CAD build for the part. Positions are in the model's coordinates, mm. Face numbers are marked on the shaded views. A direction names the side the tool comes from. Give positions to 0.01 mm unless a question says otherwise; leave off trailing zeros. Order: outer loops, then holes, each group sorted by start corner. A loop starts at its lowest first (then second) coordinate and runs counter-clockwise, first axis right, second up.
Item 1: Wall check: L1, parallel to Z at x = 152, y = 4.75; L2, parallel to Z at x = 124, y = 11.25; L3, parallel to Y at x = 95, z = 6. Give the ranges that are in metal, low to high.
Item 2: Which spindle directions (+Z, -Z, +X, -X, +Y, -Y) get a long thin tool onto all of the face, cutting with end or side? Do the marked faces 1 and 2. Say none if no direction does.
Item 3: Flat gauge pins, fed straight in: P1, Ø12, axis at x = 61.5, z = -30.5, coming from the -Y side; P2, Ø13, axis at x = 152.4, z = -25.4, coming from the +Y side; P3, Ø17.5, axis at x = 76.2, z = -25.4, coming from the +Y side. Where does each tip first touch, or does it go through?
Item 4: Band-saw the part on D-D on x = 107. Give the cut face in (y, z), plus the area to 3 significant figures.
Item 5: Two-plate mould, pull along X, no slides. Class the marked faces 3, 4, 5 and 6: released by +X, released by -X, zero draft, split by the parting line, or undercut.
Item 6: Band-saw the part on B-B on y = 10. Count the separate pieces of the cut face and the enclosed holes in it, plus the area to 3 significant figures.
Item 7: Band-saw the part on A-A on x = 25.4. Give the cut face in (y, z).
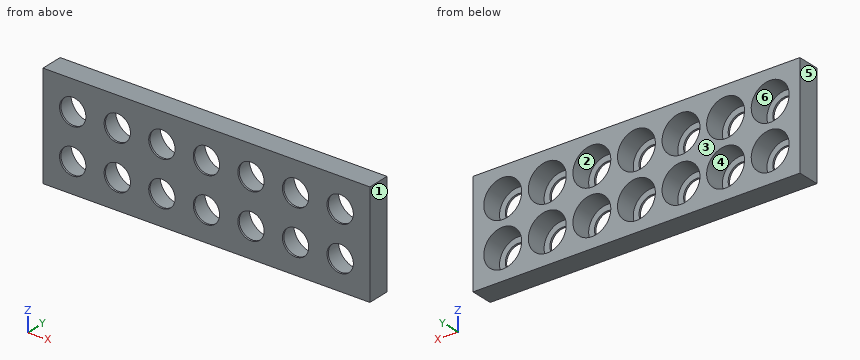
```python
from build123d import *

# Parameters (mm, degrees)
SKETCH1_W           = 186.266666666
SKETCH1_H           = 59.266666666
SKETCH1_R           = 10.8
BOSS_EXTRUDE2_DEPTH = 12.7
SKETCH1_4_R         = 10.8
SKETCH1_4_R_2       = 7.5
BOSS_EXTRUDE3_DEPTH = 1.016


with BuildPart() as part:
    # Sketch1 → Boss-Extrude2 (new body)
    with BuildSketch(Plane(origin=(0, 0, 0), x_dir=(1, 0, 0), z_dir=(0, 1, 0))):
        with Locations((76.2, 12.7)):
            Rectangle(SKETCH1_W, SKETCH1_H)
        with Locations(Location((0, 25.4, 0), (0, 0, 270))):
            Circle(SKETCH1_R, mode=Mode.SUBTRACT)
        with Locations(Location((152.4, 25.4, 0), (0, 0, 270))):
            Circle(SKETCH1_R, mode=Mode.SUBTRACT)
        with Locations(Location((127, 25.4, 0), (0, 0, 270))):
            Circle(SKETCH1_R, mode=Mode.SUBTRACT)
        with Locations(Location((101.6, 25.4, 0), (0, 0, 270))):
            Circle(SKETCH1_R, mode=Mode.SUBTRACT)
        with Locations(Location((76.2, 25.4, 0), (0, 0, 270))):
            Circle(SKETCH1_R, mode=Mode.SUBTRACT)
        with Locations(Location((50.8, 25.4, 0), (0, 0, 270))):
            Circle(SKETCH1_R, mode=Mode.SUBTRACT)
        with Locations(Location((25.4, 25.4, 0), (0, 0, 270))):
            Circle(SKETCH1_R, mode=Mode.SUBTRACT)
        with Locations(Location((152.4, 0, 0), (0, 0, 270))):
            Circle(SKETCH1_R, mode=Mode.SUBTRACT)
        with Locations(Location((127, 0, 0), (0, 0, 270))):
            Circle(SKETCH1_R, mode=Mode.SUBTRACT)
        with Locations(Location((101.6, 0, 0), (0, 0, 270))):
            Circle(SKETCH1_R, mode=Mode.SUBTRACT)
        with Locations(Location((76.2, 0, 0), (0, 0, 270))):
            Circle(SKETCH1_R, mode=Mode.SUBTRACT)
        with Locations(Location((50.8, 0, 0), (0, 0, 270))):
            Circle(SKETCH1_R, mode=Mode.SUBTRACT)
        with Locations(Location((25.4, 0, 0), (0, 0, 270))):
            Circle(SKETCH1_R, mode=Mode.SUBTRACT)
        with Locations(Location((0, 0, 0), (0, 0, 270))):
            Circle(SKETCH1_R, mode=Mode.SUBTRACT)
    extrude(amount=BOSS_EXTRUDE2_DEPTH)

    # Sketch1_4 → Boss-Extrude3 (add)
    # profile 1 of 14: a face of its own
    with BuildSketch(Plane(origin=(0, 0, 0), x_dir=(1, 0, 0), z_dir=(0, 1, 0))):
        with Locations(Location((0, 25.4, 0), (0, 0, 270))):
            Circle(SKETCH1_4_R)
        with Locations(Location((0, 25.4, 0), (0, 0, 270))):
            Circle(SKETCH1_4_R_2, mode=Mode.SUBTRACT)
    # profile 2 of 14: a face of its own
    with BuildSketch(Plane(origin=(0, 0, 0), x_dir=(1, 0, 0), z_dir=(0, 1, 0))):
        with Locations(Location((25.4, 25.4, 0), (0, 0, 270))):
            Circle(SKETCH1_4_R)
        with Locations(Location((25.4, 25.4, 0), (0, 0, 270))):
            Circle(SKETCH1_4_R_2, mode=Mode.SUBTRACT)
    # profile 3 of 14: a face of its own
    with BuildSketch(Plane(origin=(0, 0, 0), x_dir=(1, 0, 0), z_dir=(0, 1, 0))):
        with Locations(Location((50.8, 25.4, 0), (0, 0, 270))):
            Circle(SKETCH1_4_R)
        with Locations(Location((50.8, 25.4, 0), (0, 0, 270))):
            Circle(SKETCH1_4_R_2, mode=Mode.SUBTRACT)
    # profile 4 of 14: a face of its own
    with BuildSketch(Plane(origin=(0, 0, 0), x_dir=(1, 0, 0), z_dir=(0, 1, 0))):
        with Locations(Location((76.2, 25.4, 0), (0, 0, 270))):
            Circle(SKETCH1_4_R)
        with Locations(Location((76.2, 25.4, 0), (0, 0, 270))):
            Circle(SKETCH1_4_R_2, mode=Mode.SUBTRACT)
    # profile 5 of 14: a face of its own
    with BuildSketch(Plane(origin=(0, 0, 0), x_dir=(1, 0, 0), z_dir=(0, 1, 0))):
        with Locations(Location((101.6, 25.4, 0), (0, 0, 270))):
            Circle(SKETCH1_4_R)
        with Locations(Location((101.6, 25.4, 0), (0, 0, 270))):
            Circle(SKETCH1_4_R_2, mode=Mode.SUBTRACT)
    # profile 6 of 14: a face of its own
    with BuildSketch(Plane(origin=(0, 0, 0), x_dir=(1, 0, 0), z_dir=(0, 1, 0))):
        with Locations(Location((127, 25.4, 0), (0, 0, 270))):
            Circle(SKETCH1_4_R)
        with Locations(Location((127, 25.4, 0), (0, 0, 270))):
            Circle(SKETCH1_4_R_2, mode=Mode.SUBTRACT)
    # profile 7 of 14: a face of its own
    with BuildSketch(Plane(origin=(0, 0, 0), x_dir=(1, 0, 0), z_dir=(0, 1, 0))):
        with Locations(Location((152.4, 25.4, 0), (0, 0, 270))):
            Circle(SKETCH1_4_R)
        with Locations(Location((152.4, 25.4, 0), (0, 0, 270))):
            Circle(SKETCH1_4_R_2, mode=Mode.SUBTRACT)
    # profile 8 of 14: a face of its own
    with BuildSketch(Plane(origin=(0, 0, 0), x_dir=(1, 0, 0), z_dir=(0, 1, 0))):
        with Locations(Location((0, 0, 0), (0, 0, 270))):
            Circle(SKETCH1_4_R)
        with Locations(Location((0, 0, 0), (0, 0, 270))):
            Circle(SKETCH1_4_R_2, mode=Mode.SUBTRACT)
    # profile 9 of 14: a face of its own
    with BuildSketch(Plane(origin=(0, 0, 0), x_dir=(1, 0, 0), z_dir=(0, 1, 0))):
        with Locations(Location((25.4, 0, 0), (0, 0, 270))):
            Circle(SKETCH1_4_R)
        with Locations(Location((25.4, 0, 0), (0, 0, 270))):
            Circle(SKETCH1_4_R_2, mode=Mode.SUBTRACT)
    # profile 10 of 14: a face of its own
    with BuildSketch(Plane(origin=(0, 0, 0), x_dir=(1, 0, 0), z_dir=(0, 1, 0))):
        with Locations(Location((50.8, 0, 0), (0, 0, 270))):
            Circle(SKETCH1_4_R)
        with Locations(Location((50.8, 0, 0), (0, 0, 270))):
            Circle(SKETCH1_4_R_2, mode=Mode.SUBTRACT)
    # profile 11 of 14: a face of its own
    with BuildSketch(Plane(origin=(0, 0, 0), x_dir=(1, 0, 0), z_dir=(0, 1, 0))):
        with Locations(Location((76.2, 0, 0), (0, 0, 270))):
            Circle(SKETCH1_4_R)
        with Locations(Location((76.2, 0, 0), (0, 0, 270))):
            Circle(SKETCH1_4_R_2, mode=Mode.SUBTRACT)
    # profile 12 of 14: a face of its own
    with BuildSketch(Plane(origin=(0, 0, 0), x_dir=(1, 0, 0), z_dir=(0, 1, 0))):
        with Locations(Location((101.6, 0, 0), (0, 0, 270))):
            Circle(SKETCH1_4_R)
        with Locations(Location((101.6, 0, 0), (0, 0, 270))):
            Circle(SKETCH1_4_R_2, mode=Mode.SUBTRACT)
    # profile 13 of 14: a face of its own
    with BuildSketch(Plane(origin=(0, 0, 0), x_dir=(1, 0, 0), z_dir=(0, 1, 0))):
        with Locations(Location((127, 0, 0), (0, 0, 270))):
            Circle(SKETCH1_4_R)
        with Locations(Location((127, 0, 0), (0, 0, 270))):
            Circle(SKETCH1_4_R_2, mode=Mode.SUBTRACT)
    # profile 14 of 14: a face of its own
    with BuildSketch(Plane(origin=(0, 0, 0), x_dir=(1, 0, 0), z_dir=(0, 1, 0))):
        with Locations(Location((152.4, 0, 0), (0, 0, 270))):
            Circle(SKETCH1_4_R)
        with Locations(Location((152.4, 0, 0), (0, 0, 270))):
            Circle(SKETCH1_4_R_2, mode=Mode.SUBTRACT)
    extrude(amount=BOSS_EXTRUDE3_DEPTH)


solid = part.part
```
The answers:
1. L1: z = -42.33 to -36.19, -14.61 to -10.79, 10.79 to 16.93
1. L2: z = -42.33 to -35.77, -15.03 to -10.37, 10.37 to 16.93
1. L3: y = 0 to 1.02
2. face 1: +Z, -Z, +X, +Y, -Y
2. face 2: +Y
3. P1: stops at y = 0
3. P2: passes through
3. P3: stops at y = 1.02
4. outline: (0, -42.33) - (12.7, -42.33) - (12.7, -34.75) - (1.02, -34.75) - (1.02, -30.6) - (0, -30.6) - close; (0, -20.2) - (1.02, -20.2) - (1.02, -16.05) - (12.7, -16.05) - (12.7, -9.35) - (1.02, -9.35) - (1.02, -5.2) - (0, -5.2) - close; (0, 5.2) - (1.02, 5.2) - (1.02, 9.35) - (12.7, 9.35) - (12.7, 16.93) - (0, 16.93) - close
4. area: 294 mm2
5. face 3: zero draft
5. face 4: undercut
5. face 5: released by -X
5. face 6: undercut
6. separate pieces: 1
6. enclosed holes: 14
6. area: 5,910 mm2
7. outline: (0, -42.33) - (12.7, -42.33) - (12.7, -36.2) - (1.02, -36.2) - (1.02, -32.9) - (0, -32.9) - close; (0, -17.9) - (1.02, -17.9) - (1.02, -14.6) - (12.7, -14.6) - (12.7, -10.8) - (1.02, -10.8) - (1.02, -7.5) - (0, -7.5) - close; (0, 7.5) - (1.02, 7.5) - (1.02, 10.8) - (12.7, 10.8) - (12.7, 16.93) - (0, 16.93) - close
